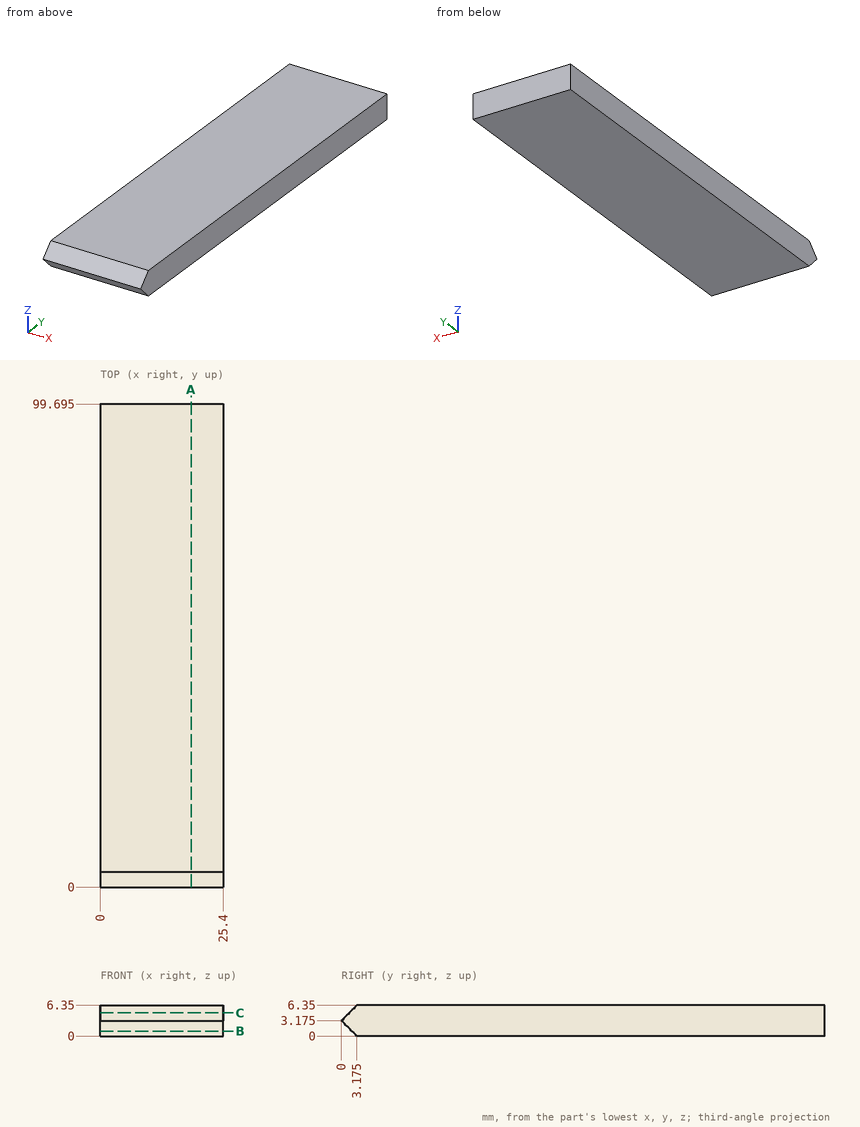
Geometry: see drawing. Coordinates: mm, zero at the bounding-box minimum. Coordinates: 2 decimals unless noted, no trailing zeros. Write each loop counter-clockwise with the first axis right and the second up, starting at its lowest first coordinate (ties: lowest second). Pieces come first, ordered by that corner, then holes.
1) Section A-A on x = 18.75. Output: boundary loops of the cut face in (y, z) (3 decimals), and give its area (3 significant figures).
2) Material intervals for line 1 along Y through (x, z) = (20.75, 5) (3 decimals); line 2 along Y through (x, z) = (7.75, 3.75) (3 decimals), sorted ascending.
3) Section B-B on z = 1. Output: boundary loops of the cut face in (x, y) (3 decimals).
4) Section C-C on z = 4.75. Output: boundary loops of the cut face in (x, y) (3 decimals).
Check result:
1. outline: (0, 3.175) - (3.175, 0) - (99.695, 0) - (99.695, 6.35) - (3.175, 6.35) - close
1. area: 623 mm2
2. line 1: y = 1.825 to 99.695
2. line 2: y = 0.575 to 99.695
3. outline: (0, 2.175) - (25.4, 2.175) - (25.4, 99.695) - (0, 99.695) - close
4. outline: (0, 1.575) - (25.4, 1.575) - (25.4, 99.695) - (0, 99.695) - close
